Verification items for the finished model (mm, model axes). Face numbers are marked on the shaded views. Coordinates: 2 decimals unless noted, no trailing zeros. Write each loop counter-clockwise with the first axis right and the second up, starting at its lowest first coordinate (ties: lowest second). Pieces come first, ordered by that corner, then holes. Notation, with made-up numbers: (57.5, 47.25) -> (106.5, 47.25) arc R22 cw to (106.5, 75.25) -> close; hole circle Ø4 at (-5, -35). An arc over 180 degrees is marked (long way). Write each question's results on one line, items separated by ' | '. Start each with the question number.
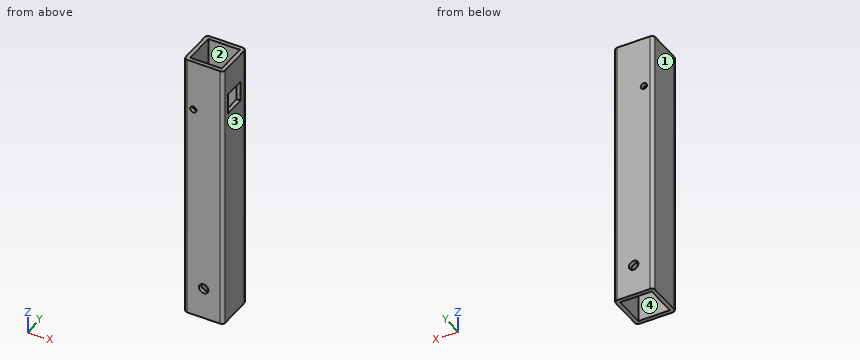
Autodesk Inventor part; units mm, degrees
ref_plane "endPlane" through (0, 0, 172.5) normal (0, 0, -1) x (-1, 0, 0)
ref_plane "midPlane" through (-10.5, -12.5, 86.25) normal (0, 0, 1) x (1, 0, 0)
ref_plane "Work Plane3" through (12.5, -7.5872, 147.5) normal (0, 0, 1) x (1, 0, 0)
sketch "Sketch1" plane through (0, 0, 0) normal (0, 0, 1) x (1, 0, 0)
  line L0 (-12.5, 12.5) -> (12.5, 12.5)
  line L1 (12.5, 12.5) -> (12.5, -12.5)
  line L2 (12.5, -12.5) -> (-12.5, -12.5)
  line L3 (-12.5, -12.5) -> (-12.5, 12.5)
  line L4 (10, 10) -> (-10, 10)
  line L5 (-10, 10) -> (-10, -10)
  line L6 (-10, -10) -> (10, -10)
  line L7 (10, -10) -> (10, 10)
  point P0 (0, 0)
  dimension "d0" = 25
  dimension "d1" = 25
  dimension "d2" = 12.5
  dimension "d3" = 12.5
  dimension "d4" = 2.5
extrude "Extrusion1" add sketch "Sketch1" along normal blind 1000
fillet "Fillet1" radius 2 4 edges at (12.5, 12.5, 500) (-12.5, 12.5, 500) (-12.5, -12.5, 500) (12.5, -12.5, 500)
ref_plane "endPlane" through (0, 0, 172.5) normal (0, 0, -1) x (-1, 0, 0)
split "Split1" plane through (0, 0, 172.5) removes the side toward (0, 0, 1)
ref_plane "midPlane" through (-10.5, -12.5, 86.25) normal (0, 0, 1) x (1, 0, 0)
sketch "Sketch2" plane through (-10.5, 12.5, 0) normal (0, 1, 0) x (1, 0, 0)
  line L0 (10.5, -20) -> (10.5, -20) construction
  line L1 (13.5, -20) -> (13.5, -20)
  line L2 (7.5, -20) -> (7.5, -20)
  arc A0 (7.5, -20) -> (13.5, -20) centre (10.5, -20) ccw
  arc A1 (13.5, -20) -> (7.5, -20) centre (10.5, -20) ccw
  point P0 (10.5, 0)
  point P1 (10.5, -40)
  dimension "d46" = 6
  dimension "d47" = 0
  dimension "d48" = 20
  dimension "d49" = 0
sketch "Sketch3" plane through (12.5, -10.5, 0) normal (1, 0, 0) x (0, 0, -1)
  line L0 (-154, 16.9128) -> (-141, 16.9128)
  line L1 (-141, 16.9128) -> (-141, 2.9128)
  line L2 (-141, 2.9128) -> (-154, 2.9128)
  line L3 (-154, 2.9128) -> (-154, 16.9128)
  line L4 (-172.5, 21) -> (-172.5, 0)
  point P0 (0, 10.5)
  dimension "d28" = 14
  dimension "d29" = 18.5
  dimension "d30" = 13
extrude "Extrusion2" cut sketch "Sketch3" against normal up to surface (2.5 mm away)
sketch "Sketch4" plane through (-10.5, 12.5, 0) normal (0, 1, 0) x (1, 0, 0)
  line L0 (-2, 0) -> (-2, -1000)
  line L1 (0, -172.5) -> (21, -172.5)
  point P0 (10.5, 0)
  point P1 (-2, -172.5)
  point P2 (4, -140)
  point P3 (23, -141)
  dimension "d36" = 6
  dimension "d45" = 1
hole "Hole2" at (-6.5, 12.5, 140) direction (0, -1, 0) diameter 4 end through all
ref_plane "Work Plane3" through (12.5, -7.5872, 147.5) normal (0, 0, 1) x (1, 0, 0)
extrude "Extrusion3" cut sketch "Sketch2" against normal through all
equation "\"d0\" = -2 * a + sm_varx_squareBarDimension - tol"
equation "\"d1\" = d0"
equation "\"d4\" = sm_varx_squareBarThickness"
equation "\"d8\" = -sm_varx_z - 0.5 * d0"
equation "\"sm_varx_squareBarThickness\" = 2.5"
equation "\"sm_varx_pinPlate_holeDiameter\" = 5"
equation "\"sm_varx_member_tolerance\" = 0"
equation "\"a\" = sm_varx_squareBarThickness"
equation "\"hoop_angle_z\" = 45deg"
equation "\"hoop_bearing_length\" = 5deg"
equation "\"hoop_cable_diam\" = 5"
equation "\"hoop_cable_pulley_diam\" = 22"
equation "\"hoop_thickness_large\" = 4"
equation "\"hoop_thickness_medium\" = 3.2"
equation "\"hoop_thickness_small\" = 2"
equation "\"hoop_width_large\" = 51"
equation "\"hoop_width_medium\" = 33.7"
equation "\"hoop_width_small\" = 25.4"
equation "\"rack_tooth_addendum\" = 5"
equation "\"rack_tooth_dedendum\" = 5"
equation "\"rack_tooth_thickness\" = 5"
equation "\"secure_arm_angle\" = 35deg"
equation "\"secure_arm_radii\" = 9"
equation "\"support_baseClamp_platformLengthBuffer\" = 35"
equation "\"support_baseClamp_platformThickness\" = 15"
equation "\"support_baseClamp_platformWidthBuffer\" = 0"
equation "\"support_baseClamp_sleeveHoleDiameter\" = 12"
equation "\"support_baseClamp_sleeveSweepTerminationAngle\" = 55deg"
equation "\"support_baseClamp_thickness\" = 8"
equation "\"support_frame_endHoleBuffer\" = 45"
equation "\"support_frame_squareBarFillet\" = 2"
equation "\"support_frame_squareBarThickness\" = 5"
equation "\"hoop_tabs_thickness\" = 6"
equation "\"hoop_tabs_hole\" = 12"
equation "\"wheelchair_deployed_width\" = 635"
equation "\"wheelchair_deployed_length\" = 1067"
equation "\"wheelchair_deployed_height\" = 914"
equation "\"sm_varx_pinPlate_thickness\" = 5"
equation "\"hoop_bushing12_radialInterference\" = 0"
equation "\"hoop_bushing23_radialInterference\" = 0"
equation "\"hoop_bushing23_od\" = -2 * hoop_thickness_medium + hoop_width_medium + hoop_bushing23_radialInterference"
equation "\"hoop_bushing23_thickness\" = -hoop_width_small + hoop_bushing23_od - 2 * hoop_bushing23_radialInterference"
equation "\"hoop_bushing12_od\" = -2 * hoop_thickness_large + hoop_width_large + hoop_bushing12_radialInterference"
equation "\"wheelchatir_pos_deploy_angle_0\" = 65deg"
equation "\"wheelchatir_pos_store_angle_0\" = 90deg"
equation "\"wheelchatir_pos_deploy_angle_1\" = 20deg"
equation "\"wheelchatir_pos_store_angle_1\" = 20deg"
equation "\"hoop_bushing12_thickness\" = -hoop_width_medium + hoop_bushing12_od - 2 * hoop_bushing12_radialInterference"
properties part number "member_transverse_inner" material "Steel, Galvanized"
1. Sectioned sample at A-A on y = -1. Record the cut outline in (x, z).
2. Sectioned sample at C-C on z = 20. Record the cut outline in (x, y).
3. Sectioned sample at D-D on x = -6.5. Record the cut outline in (y, z).
4. Depth check by flat-ended pin: pin 1 Ø12 at (x, y) = (1.5, -1) entering from +Z. Enter the tip coordinate at first touch or a pass-through.
5. Sectioned sample at B-B on x = 8.25. Record the cut outline in (y, z), plus the area to 4 significant figures.
6. Material ranges on probe 1 along Z at (x, y) = (-6.5, -10.95); probe 2 along X at (y, z) = (-3.5, 113), recorded low to high. Write a range as from..to.
7. Mould release check, pull along X, two halves, no side actions. Record for the marked faces 1, 2, 3 and 4: +X half, -X half, draft (parallel to the pull), parting line (faces both ways), or undercut.
Computed values:
1) outline: (-12.5, 0) -> (-10, 0) -> (-10, 172.5) -> (-12.5, 172.5) -> close; (10, 0) -> (12.5, 0) -> (12.5, 141) -> (10, 141) -> close; (10, 154) -> (12.5, 154) -> (12.5, 172.5) -> (10, 172.5) -> close
2) outline: (-12.5, -10.5) arc R2 ccw to (-10.5, -12.5) -> (-3, -12.5) -> (-3, -10) -> (-10, -10) -> (-10, 10) -> (-3, 10) -> (-3, 12.5) -> (-10.5, 12.5) arc R2 ccw to (-12.5, 10.5) -> close; (3, -12.5) -> (10.5, -12.5) arc R2 ccw to (12.5, -10.5) -> (12.5, 10.5) arc R2 ccw to (10.5, 12.5) -> (3, 12.5) -> (3, 10) -> (10, 10) -> (10, -10) -> (3, -10) -> close
3) outline: (-12.5, 0) -> (-10, 0) -> (-10, 138) -> (-12.5, 138) -> close; (-12.5, 142) -> (-10, 142) -> (-10, 172.5) -> (-12.5, 172.5) -> close; (10, 0) -> (12.5, 0) -> (12.5, 138) -> (10, 138) -> close; (10, 142) -> (12.5, 142) -> (12.5, 172.5) -> (10, 172.5) -> close
4) pin 1: passes through
5) outline: (-12.5, 0) -> (-10, 0) -> (-10, 172.5) -> (-12.5, 172.5) -> close; (10, 0) -> (12.5, 0) -> (12.5, 172.5) -> (10, 172.5) -> close | area: 862.5 mm^2
6) probe 1: z = 0..138, 142..172.5 | probe 2: x = -12.5..-10, 10..12.5
7) face 1: -X half | face 2: undercut | face 3: +X half | face 4: undercut
